Input: part model. Units: mm. Frame: model coordinates. A direction names the side the tool comes from. Coordinates: 2 decimals unless noted, no trailing zeros. Loops run counter-clockwise (first coordinate to the right, second up) from the corner with the lowest first, then second, coordinate; pieces in that order, holes last. Notation, with made-up numbers: (45, -8.5) -> (74, -8.5) arc R19 ccw to (74, 24.5) -> close; hole circle Ø5 at (8.25, -0.75). An arc over 180 degrees is marked (long way). Put each result on its own line as item: value. Start each with the question number.
1) Cut plane A-A (x = 0). Return the cut outline in (y, z), plus the area to 3 significant figures.
2) Cut plane B-B (z = -3.5). Return the cut outline in (x, y), plus the area to 3 significant figures.
3) Cut plane C-C (y = 12.75). Return the cut outline in (x, z), plus the area to 3 significant figures.
4) Contact query for flat-ended pins moving along their axis: P1, Ø1, axis at x = -1, z = 7, coming from the +Y side; P2, Ø7, axis at x = -1, z = 16.5, coming from the -Y side; P3, Ø1.7, axis at x = 0, z = 12.5, coming from the -Y side; P4, Ø6, axis at x = 1, y = 3.5, coming from the +Z side (3 decimals). Output: stop coordinate, or through.
5) Pull-direction query (X, two-part tool) for faces 1 (the flat face through (7.5, 11, -2)), 2 (the flat face through (0, 11, 18)), 3 (the flat face through (-6.7, 12.2, 18.8)); classes: pulls with the +X half, pulls with the -X half, needs draft (parallel to the pull), parting line crosses it, or undercut.
6) Material intervals for L1, parallel to X at y = 10.15, z = 12.5; L2, parallel to Y at x = 6, z = 12; L3, parallel to Z at x = 1, y = 13.25, sorted ascending.
7) Set-up query: faces 4 (the cylindrical face through (0.027, 9.479, 11.536)), 5 (the cylindrical face through (0.05, 8.18, -9.25)), 6 (the flat face through (0, 8, 11)), 7 (the flat face through (-7.5, 11, -2)), 8 (the flat face through (3.8, 9.5, 16.3)). Return all of +Z, -Z, +X, -X, +Y, -Y with unobstructed straight access to the full face (end or side cutting, diameter ignored); none if empty.
8) Cut plane D-D (z = 12.5). Return the cut outline in (x, y), plus the area to 3 significant figures.
from build123d import *

# Parameters (mm, degrees)
SKETCH1_W           = 15
SKETCH1_H           = 40
BOSS_EXTRUDE1_DEPTH = 15
CUT_EXTRUDE1_DEPTH  = 30.154759474
FILLET1_R           = 15
CUT_EXTRUDE2_DEPTH  = 3
FILLET2_R           = 0.5
FILLET4_R           = 0.5
CHAMFER1_SIZE       = 2
FILLET6_R           = 5
CUT_EXTRUDE3_DEPTH  = 27.100766272


with BuildPart() as part:
    # Sketch1 → Boss-Extrude1 (new body)
    with BuildSketch(Plane(origin=(0, 0, 0), x_dir=(1, 0, 0), z_dir=(0, 1, 0))):
        Rectangle(SKETCH1_W, SKETCH1_H)
    extrude(amount=BOSS_EXTRUDE1_DEPTH)

    # Sketch3 → Cut-Extrude1 (cut, through all)
    with BuildSketch(Plane.ZY.offset(7.5)):
        Polygon((20, 0), (20, 8), (-5.121506718, 8), (-9.96820088, 0), align=None)
    extrude(amount=-CUT_EXTRUDE1_DEPTH, mode=Mode.SUBTRACT)

    # Fillet1
    fillet1_edges = [part.edges().sort_by_distance(p)[0] for p in [
        (0, 8, -5.121506718),
    ]]
    fillet(fillet1_edges, radius=FILLET1_R)

    # Sketch5 → Cut-Extrude2 (cut)
    with BuildSketch(Plane.XZ.offset(-8)):
        with BuildLine():
            Line((7.5, 20), (0.681678783, 13.181678783))
            ThreePointArc((0.681678783, 13.181678783), (0, 11.53596062), (-0.681678783, 13.181678783))
            Line((-0.681678783, 13.181678783), (-7.5, 20))
            Line((-7.5, 20), (7.5, 20))
        make_face()
    extrude(amount=-CUT_EXTRUDE2_DEPTH, mode=Mode.SUBTRACT)

    # Fillet2
    fillet2_edges = [part.edges().sort_by_distance(p)[0] for p in [
        (0.681678783, 9.5, 13.181678783),
        (-0.681678783, 9.5, 13.181678783),
    ]]
    fillet(fillet2_edges, radius=FILLET2_R)

    # Fillet4
    fillet4_edges = [part.edges().sort_by_distance(p)[0] for p in [
        (-7.5, 9.5, 20),
        (7.5, 9.5, 20),
    ]]
    fillet(fillet4_edges, radius=FILLET4_R)

    # Chamfer1
    # the kernel refuses this chamfer: 2 mm, written as the material it takes off along each edge
    with BuildSketch(Plane(origin=(7.5, 5.856634024, 20), x_dir=(0.02749587661058651, 0, -0.9996219169112968), z_dir=(0, 1, 0))) as chamfer1_piece_1:
        Polygon((CHAMFER1_SIZE * 0.999621916911, CHAMFER1_SIZE * 0.0274958766106), (-CHAMFER1_SIZE * 0.0274958766106, CHAMFER1_SIZE * 0.999621916911), (0, 0), align=None)
    extrude(amount=14.286731952, mode=Mode.SUBTRACT)
    with BuildSketch(Plane(origin=(-7.5, 5.856634024, 20), x_dir=(-0.02749587661058651, 0, -0.9996219169112968), z_dir=(0, 1, 0))) as chamfer1_piece_2:
        Polygon((CHAMFER1_SIZE * 0.999621916911, -CHAMFER1_SIZE * 0.0274958766106), (-CHAMFER1_SIZE * 0.0274958766106, -CHAMFER1_SIZE * 0.999621916911), (0, 0), align=None)
    extrude(amount=14.286731952, mode=Mode.SUBTRACT)

    # Fillet6
    fillet6_edges = [part.edges().sort_by_distance(p)[0] for p in [
        (-7.5, 7.5, -20),
        (7.5, 7.5, -20),
    ]]
    fillet(fillet6_edges, radius=FILLET6_R)

    # Sketch6 → Cut-Extrude3 (cut, through all)
    with BuildSketch(Plane(origin=(0, 15, 0), x_dir=(1, 0, 0), z_dir=(0, 1, 0))):
        with BuildLine():
            Line((-2.25, 7), (-2.25, -8.056468678))
            ThreePointArc((-2.25, -8.056468678), (0, -10.306468678), (2.25, -8.056468678))
            Line((2.25, -8.056468678), (2.25, 7))
            ThreePointArc((2.25, 7), (0, 9.25), (-2.25, 7))
        make_face()
    extrude(amount=-CUT_EXTRUDE3_DEPTH, mode=Mode.SUBTRACT)


solid = part.part
Results found:
1. outline: (0, -20) -> (15, -20) -> (15, -9.25) -> (1.17, -9.25) arc R15 cw to (0.77, -9.5) -> (0, -9.97) -> close; (8, 10.31) -> (15, 10.31) -> (15, 20) -> (11, 20) -> (11, 11.54) -> (8, 11.54) -> close
1. area: 203 mm2
2. outline: (-7.5, 6.36) -> (-2.25, 6.36) -> (-2.25, 15) -> (-7.5, 15) -> close; (2.25, 6.36) -> (7.5, 6.36) -> (7.5, 15) -> (2.25, 15) -> close
2. area: 90.8 mm2
3. outline: (-7.5, -15) arc R5 ccw to (-2.5, -20) -> (2.5, -20) arc R5 ccw to (7.5, -15) -> (7.5, 18) -> (5.5, 20) -> (-5.5, 20) -> (-7.5, 18) -> close; hole (-2.25, -7) arc R2.25 ccw to (2.25, -7) -> (2.25, 8.06) arc R2.25 ccw to (-2.25, 8.06) -> close
3. area: 502 mm2
4. P1: passes through
4. P2: stops at y = 8
4. P3: stops at y = 11
4. P4: stops at z = -3.745
5. face 1: pulls with the +X half
5. face 2: undercut
5. face 3: pulls with the -X half
6. L1: x = -7.5 to -0.96, 0.96 to 7.5
6. L2: y = 8 to 15
6. L3: z = -20 to -9.02, 10.07 to 20
7. face 4: -Y
7. face 5: +Y, -Y
7. face 6: +Z, +X, -X, -Y
7. face 7: +Z, -Z, -X, +Y, -Y
7. face 8: +Z, -Y
8. outline: (-7.5, 8) -> (-0.96, 8) -> (-0.96, 11) -> (0.96, 11) -> (0.96, 8) -> (7.5, 8) -> (7.5, 15) -> (-7.5, 15) -> close
8. area: 99.2 mm2
